Input: part model. Units: mm. Frame: model coordinates. Face numbers are marked on the shaded views. A direction names the side the tool comes from. Coordinates: 2 decimals unless noted, no trailing zeros. Loops run counter-clockwise (first coordinate to the right, second up) from the corner with the lowest first, then second, coordinate; pieces in that order, holes last. Notation, with made-up numbers: (29.25, 83) - (79.25, 83) arc R5 ccw to (79.25, 87) - close; hole circle Ø3 at (49.5, 24.5). An arc over 180 degrees is marked (long way). Use one line per item in the form item = value.
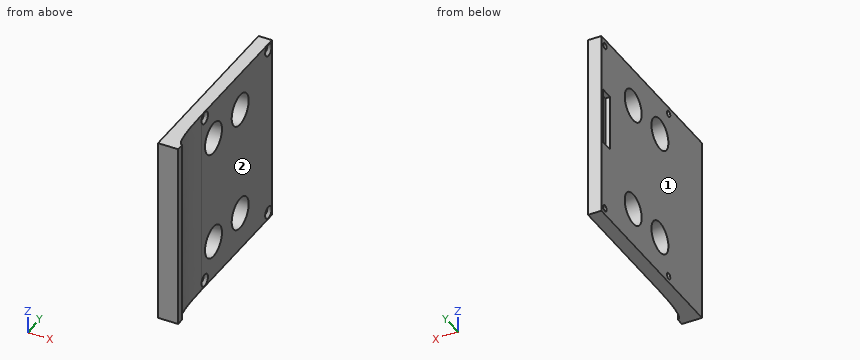
from build123d import *

# Parameters (mm, degrees)
BOSS_EXTRUDE1_DEPTH                            = 98
SKETCH2_R                                      = 8.25
CUT_EXTRUDE1_DEPTH                             = 114.573245575
CSK_FOR_M3_FLAT_HEAD_MACHINE_SCREW2_AT_2_COUNT = 2
CSK_FOR_M3_FLAT_HEAD_MACHINE_SCREW2_AT_2_PITCH = 62
CSK_FOR_M3_FLAT_HEAD_MACHINE_SCREW2_AT_3_COUNT = 2
CSK_FOR_M3_FLAT_HEAD_MACHINE_SCREW2_AT_3_PITCH = 110.113577728
CSK_FOR_M3_FLAT_HEAD_MACHINE_SCREW2_AT_4_COUNT = 2
CSK_FOR_M3_FLAT_HEAD_MACHINE_SCREW2_AT_4_PITCH = 91
SKETCH9_W                                      = 29.5
SKETCH9_H                                      = 7
CUT_EXTRUDE2_DEPTH                             = 2.5


with BuildPart() as part:
    # Sketch1 → Boss-Extrude1 (new body)
    with BuildSketch(Plane.XY):
        with BuildLine():
            Line((-46.838690812, 41.567455511), (-46.838690812, -56.432544489))
            Line((-46.838690812, -56.432544489), (-36.338690812, -56.432544489))
            Line((-36.338690812, -56.432544489), (-36.338690812, -52.432544489))
            add(Edge.make_bspline(
                [(-39.838690812, -26.932544489), (-39.838690812, -52.432544489), (-36.338690812, -52.432544489)],
                knots=[0, 0, 0, 1, 1, 1], degree=2))
            Line((-39.838690812, -26.932544489), (-39.838690812, 41.567455511))
            Line((-39.838690812, 41.567455511), (-46.838690812, 41.567455511))
        make_face()
    extrude(amount=BOSS_EXTRUDE1_DEPTH)

    # Sketch2 → Cut-Extrude1 (cut, through all)
    with BuildSketch(Plane.ZY.offset(46.838690812)):
        with Locations((20, 10.567455511)):
            Circle(SKETCH2_R)
        with Locations((78, 10.567455511)):
            Circle(SKETCH2_R)
        with Locations((78, -15.432544489)):
            Circle(SKETCH2_R)
        with Locations((20, -15.432544489)):
            Circle(SKETCH2_R)
    extrude(amount=-CUT_EXTRUDE1_DEPTH, mode=Mode.SUBTRACT)

    # Sketch8 → CSK for M3 Flat Head Machine Screw2 (revolve, cut)
    with BuildSketch(Plane(origin=(-39.838690812, 38.067455511, 94.5), x_dir=(0, 0, -1), z_dir=(0, 1, 0))):
        Polygon((0, 0), (0, 10.96137699), (1.6, 10), (1.6, 1.55), (3.15, 0), align=None)
    csk_for_m3_flat_head_machine_screw2 = revolve(axis=Axis((-33.488690812, 38.067455511, 94.5), (-1, 0, 0)), mode=Mode.SUBTRACT)

    # CSK for M3 Flat Head Machine Screw2 at 2: CSK for M3 Flat Head Machine Screw2 ×2
    with Locations(*[(0, -i * CSK_FOR_M3_FLAT_HEAD_MACHINE_SCREW2_AT_2_PITCH, 0) for i in range(1, CSK_FOR_M3_FLAT_HEAD_MACHINE_SCREW2_AT_2_COUNT)]):
        add(csk_for_m3_flat_head_machine_screw2, mode=Mode.SUBTRACT)

    # CSK for M3 Flat Head Machine Screw2 at 3: CSK for M3 Flat Head Machine Screw2 ×2
    with Locations(*[Vector(0, -0.5630549953912599, -0.8264194287194296) * (i * CSK_FOR_M3_FLAT_HEAD_MACHINE_SCREW2_AT_3_PITCH) for i in range(1, CSK_FOR_M3_FLAT_HEAD_MACHINE_SCREW2_AT_3_COUNT)]):
        add(csk_for_m3_flat_head_machine_screw2, mode=Mode.SUBTRACT)

    # CSK for M3 Flat Head Machine Screw2 at 4: CSK for M3 Flat Head Machine Screw2 ×2
    with Locations(*[(0, 0, -i * CSK_FOR_M3_FLAT_HEAD_MACHINE_SCREW2_AT_4_PITCH) for i in range(1, CSK_FOR_M3_FLAT_HEAD_MACHINE_SCREW2_AT_4_COUNT)]):
        add(csk_for_m3_flat_head_machine_screw2, mode=Mode.SUBTRACT)

    # Sketch9 → Cut-Extrude2 (cut)
    with BuildSketch(Plane.ZY.offset(46.838690812)):
        with Locations((54.25, 36.567455511)):
            Rectangle(SKETCH9_W, SKETCH9_H)
    extrude(amount=-CUT_EXTRUDE2_DEPTH, mode=Mode.SUBTRACT)


solid = part.part
Q1. Cut plane A-A, the plane y = -18.5. Return loops of the section in (x, z).
Check values:
outline = (-46.84, 0) - (-39.84, 0) - (-39.84, 12.34) - (-46.84, 12.34) - close; (-46.84, 27.66) - (-39.84, 27.66) - (-39.84, 70.34) - (-46.84, 70.34) - close; (-46.84, 85.66) - (-39.84, 85.66) - (-39.84, 98) - (-46.84, 98) - close
Q2. First-contact query: P1, Ø2, axis at y = 19.5, z = 41.5, coming from the +X side; P2, Ø4, axis at y = 38.07, z = 3.5, coming from the +X side; P3, Ø3.5, axis at y = 35.5, z = 56.5, coming from the -X side; P4, Ø5, axis at x = -39, z = 32.5, coming from the +Y side. Flat tips, straight axial feed; report the tip coordinate or a pass-through.
Check values:
P1 = -39.84
P2 = -40.99
P3 = -44.34
P4 = 41.57
Q3. Set-up query: the marked faces 1 and 2. Return all of +Z, -Z, +X, -X, +Y, -Y with unobstructed straight access to the full face (end or side cutting, diameter ignored); none if empty.
Check values:
face_1 = +Z, -Z, -X, +Y, -Y
face_2 = +Z, -Z, +X, +Y
Q4. Cut plane D-D, the plane y = 17. Return loops of the section in (x, z).
Check values:
outline = (-46.84, 0) - (-39.84, 0) - (-39.84, 14.83) - (-46.84, 14.83) - close; (-46.84, 25.17) - (-39.84, 25.17) - (-39.84, 72.83) - (-46.84, 72.83) - close; (-46.84, 83.17) - (-39.84, 83.17) - (-39.84, 98) - (-46.84, 98) - close
Q5. Ray query, line 1 along Y through (x, z) = (-43.75, 78.5); line 2 along Y through (x, z) = (-44.8, 3.5); line 3 along Z through (x, y) = (-43.5, -19). Return the intervals inside material, ascending. Write a range as [from, to].
Check values:
line_1 = [-56.43, -23.67], [-7.2, 2.33], [18.8, 41.57]
line_2 = [-56.43, -25.53], [-22.33, 36.47], [39.67, 41.57]
line_3 = [0, 12.56], [27.44, 70.56], [85.44, 98]
Q6. Cut plane B-B, the plane z = 78. Give the number of separate pieces and of enclosed holes in the cut face, then the cut area to 3 significant figures.
Check values:
separate_pieces = 3
enclosed_holes = 0
area = 484 mm²
